Source: CAD feature listing. Evaluate the final solid. Frame: model axes, mm. Face numbers are marked on the shaded views. A direction names the side the tool comes from. Coordinates: 2 decimals unless noted, no trailing zeros. Order: outer loops, then holes, each group sorted by start corner. A loop starts at its lowest first (then second) coordinate and runs counter-clockwise, first axis right, second up.
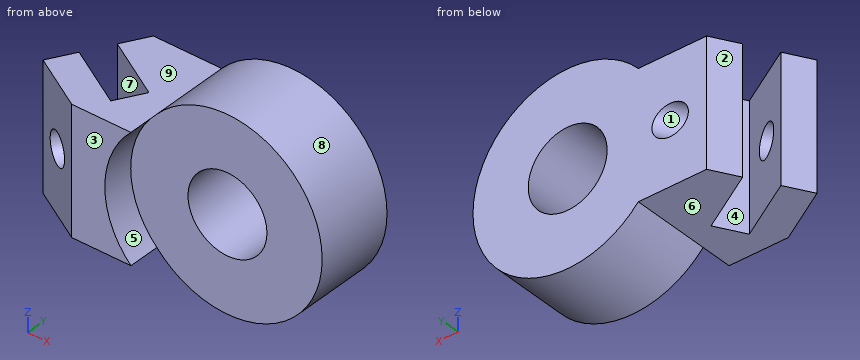
```python
from build123d import *

# Parameters (mm, degrees)
SKETCH_2_R               = 6
EXTRUDE_1_DEPTH          = 5
SKETCH_3_R               = 2.5
CUT_EXTRUDE_1_DEPTH      = 5
SKETCH_4_W               = 8.617209121
SKETCH_4_H               = 5
EXTRUDE_2_DEPTH          = 4
SKETCH_5_W               = 17.690730237
SKETCH_5_H               = 8.258947269
CUT_EXTRUDE_3_DEPTH      = 4.5
EXTRUDE_5_DEPTH          = 2
CUT_EXTRUDE_7_DEPTH      = 1
CUT_EXTRUDE_7_DEPTH_BACK = 1
SKETCH_10_W              = 4.403388768
SKETCH_10_H              = 8
CUT_EXTRUDE_8_DEPTH      = 4
SKETCH_15_R              = 1
CUT_EXTRUDE_9_DEPTH      = 8


with BuildPart() as part:
    # 草图2 → 凸台-拉伸1 (new body)
    with BuildSketch(Plane(origin=(0, 0, 0), x_dir=(1, 0, 0), z_dir=(0, 1, 0))):
        with Locations(Location((0, 0, 0), (0, 0, 270))):
            Circle(SKETCH_2_R)
    extrude(amount=EXTRUDE_1_DEPTH)

    # 草图3 → 切除-拉伸1 (cut)
    with BuildSketch(Plane(origin=(0, 5, 0), x_dir=(1, 0, 0), z_dir=(0, 1, 0))):
        with Locations(Location((0, 0, 0), (0, 0, 270))):
            Circle(SKETCH_3_R)
    extrude(amount=-CUT_EXTRUDE_1_DEPTH, mode=Mode.SUBTRACT)

    # 草图4 → 凸台-拉伸2 (add, symmetric)
    with BuildSketch(Plane.XY):
        with Locations((-7.378700456, 2.5)):
            Rectangle(SKETCH_4_W, SKETCH_4_H)
    extrude(amount=EXTRUDE_2_DEPTH, both=True)

    # 草图5 → 切除-拉伸3 (cut)
    with BuildSketch(Plane(origin=(-8.765478763, 5.060751523, 0), x_dir=(0, 0, 1), z_dir=(0.8660254037844398, -0.499999999999998, 0))):
        with Locations((1.152187915, 4.129473635)):
            Rectangle(SKETCH_5_W, SKETCH_5_H)
    extrude(amount=-CUT_EXTRUDE_3_DEPTH, mode=Mode.SUBTRACT)

    # 草图12 → 凸台-拉伸5 (add)
    with BuildSketch(Plane.XZ):
        with BuildLine():
            Line((-11.687305017, 4), (-4.472135955, 4))
            ThreePointArc((-4.472135955, 4), (-6.128990204, 0), (-4.472135955, -4))
            Line((-4.472135955, -4), (-11.687305017, -4))
            Line((-11.687305017, -4), (-11.687305017, 4))
        make_face()
    extrude(amount=EXTRUDE_5_DEPTH)

    # 草图10 → 切除-拉伸7 (cut, two sides: drawn at the far end of the back side and taken through both)
    with BuildSketch(Plane(origin=(-1.478450581, -2.560751523, 0), x_dir=(0.8660254037844398, -0.49999999999999806, 0), z_dir=(0.499999999999998, 0.8660254037844397, 0)).offset(-CUT_EXTRUDE_7_DEPTH_BACK)):
        with Locations((-7.919808662, 0)):
            Rectangle(SKETCH_10_W, SKETCH_10_H)
    extrude(amount=CUT_EXTRUDE_7_DEPTH + CUT_EXTRUDE_7_DEPTH_BACK, mode=Mode.SUBTRACT)

    # 草图14 → 切除-拉伸8 (cut)
    with BuildSketch(Plane(origin=(-2.921826254, -5.060751523, 0), x_dir=(0.8660254037844398, -0.499999999999998, 0), z_dir=(0.49999999999999806, 0.8660254037844399, 0))):
        Polygon((-9.121503046, 4), (-5.535941973, 4), (-5.535941973, -4), (-9.121503046, -4), (-10.121503046, -4), (-10.121503046, 4), align=None)
    extrude(amount=-CUT_EXTRUDE_8_DEPTH, mode=Mode.SUBTRACT)

    # 草图15 → 切除-拉伸9 (cut)
    with BuildSketch(Plane(origin=(-2.921826254, -5.060751523, 0), x_dir=(0.8660254037844397, -0.4999999999999983, 0), z_dir=(-0.4999999999999982, -0.8660254037844396, 0))):
        with Locations((-8.121503046, 0)):
            Circle(SKETCH_15_R)
    extrude(amount=-CUT_EXTRUDE_9_DEPTH, mode=Mode.SUBTRACT)


solid = part.part
```
Q1. Section query A-A on x = 0. Output: boundary loops of the cut face in (y, z), plus the area to 3 significant figures.
Solutions:
outline: (0, -6) - (5, -6) - (5, -2.5) - (0, -2.5) - close; (0, 2.5) - (5, 2.5) - (5, 6) - (0, 6) - close
area: 35.0 mm2
Q2. Set-up query: the marked faces 5, 6, 7, 8 and 9. Return all of +Z, -Z, +X, -X, +Y, -Y with unobstructed straight access to the full face (end or side cutting, diameter ignored); none if empty.
Solutions:
face 5: +X, -Y
face 6: -Z, -X, +Y, -Y
face 7: +Z, -Z
face 8: +Y, -Y
face 9: +Z, -X, +Y, -Y
Q3. Section query C-C on z = 0. Output: boundary loops of the cut face in (x, y), plus the area to 3 significant figures.
Solutions:
outline: (-11.69, 0) - (-10.82, -0.5) - (-9.88, 1.13) - (-10.74, 1.63) - close; (-9.74, 3.37) - (-8.88, 2.87) - (-7.65, 5) - (-8.8, 5) - close; (-9.09, -1.5) - (-8.22, -2) - (-6.13, -2) - (-6.13, 0) - (-2.5, 0) - (-2.5, 5) - (-5.34, 5) - (-7.15, 1.87) - (-5.93, 1.16) - (-6.93, -0.57) - (-8.15, 0.13) - close; (2.5, 0) - (6, 0) - (6, 5) - (2.5, 5) - close
area: 45.2 mm2
Q4. Material intervals for line 1 along Y through (x, z) = (-3, -1.5); line 2 along X through (y, z) = (1.3, 0); line 3 along X through (y, z) = (4.5, -2.25), sorted ascending.
Solutions:
line 1: y = 0 to 5
line 2: x = -10.94 to -10.17, -6.17 to -2.5, 2.5 to 6
line 3: x = -9.09 to -1.09, 1.09 to 5.56
Q5. Pin query (flat end, axial travel): P1, Ø6, axis at x = -1, z = -1, coming from the -Y side. Return the tip coordinate at first contact, or that it passes through.
Solutions:
P1: stops at y = 0
Q6. Section query D-D on z = 1.25. Output: boundary loops of the cut face in (x, y).
Solutions:
outline: (-11.69, 0) - (-8.22, -2) - (-5.99, -2) - (-5.99, 0) - (-2.17, 0) - (-2.17, 5) - (-8.8, 5) - (-9.74, 3.37) - (-5.93, 1.16) - (-6.93, -0.57) - (-10.74, 1.63) - close; (2.17, 0) - (5.87, 0) - (5.87, 5) - (2.17, 5) - close
Q7. Section query B-B on z = -1.5. Output: boundary loops of the cut face in (x, y), plus the area to 3 significant figures.
Solutions:
outline: (-11.69, 0) - (-8.22, -2) - (-5.93, -2) - (-5.93, 0) - (-2, 0) - (-2, 5) - (-8.8, 5) - (-9.74, 3.37) - (-5.93, 1.16) - (-6.93, -0.57) - (-10.74, 1.63) - close; (2, 0) - (5.81, 0) - (5.81, 5) - (2, 5) - close
area: 59.5 mm2
Q8. Pull-direction query (Y, two-part tool) for the marked faces 1, 2, 3 and 4; classes: pulls with the +Y half, pulls with the -Y half, needs draft (parallel to the pull), parting line crosses it, or undercut.
Solutions:
face 1: undercut
face 2: pulls with the +Y half
face 3: pulls with the -Y half
face 4: undercut
